Check sheet for the modelled part. Datum: model origin and axes. Units: mm. Face numbers are marked on the shaded views. A direction names the side the tool comes from. Coordinates: 2 decimals unless noted, no trailing zeros. Write each loop counter-clockwise with the first axis right and the second up, starting at its lowest first coordinate (ties: lowest second). Pieces come first, ordered by that corner, then holes. Notation, with made-up numbers: (9.5, -13) - (56.5, -13) arc R19 ccw to (56.5, 21) - close; hole circle Ø3 at (54.25, -20.5). An arc over 180 degrees is marked (long way). Write each question's results on one line, items separated by ' | '.
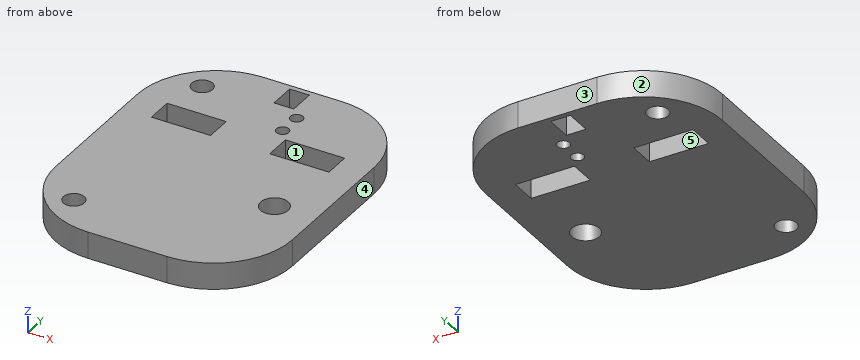
Autodesk Inventor part; units mm, degrees
ref_plane "YZ Plane" through (0, 0, 0) normal (1, 0, 0) x (0, 1, 0)
ref_plane "XZ Plane" through (0, 0, 0) normal (0, 1, 0) x (-1, 0, 0)
ref_plane "XY Plane" through (0, 0, 0) normal (0, 0, 1) x (1, 0, 0)
sketch "Sketch1" plane through (0, 0, 0) normal (0, 0, 1) x (1, 0, 0)
  circle A0 centre (10.5, 65) radius 2.65
  circle A1 centre (10.5, 10) radius 2.65
  circle A2 centre (49.5, 30) radius 3.5
  line L0 (60, 75) -> (60, 0)
  line L1 (60, 0) -> (0, 0)
  line L2 (0, 0) -> (0, 75)
  line L3 (0, 75) -> (60, 75)
  point P0 (30, 75)
  dimension "d0" = 39
  dimension "d1" = 5.3
  dimension "d2" = 55
  dimension "d3" = 10
  dimension "d5" = 10.5
  dimension "d16" = 10.5
  dimension "d19" = 20
  dimension "d22" = 7
  dimension "d55" = 75
  dimension "d64" = 60
extrude "Extrusion1" add sketch "Sketch1" along normal blind 6.731
sketch "Sketch3" plane through (0, 0, 6.731) normal (0, 0, 1) x (1, 0, 0)
  line L0 (60, 0) -> (60, 75)
  line L1 (60, 75) -> (0, 75)
  line L2 (0, 75) -> (0, 0)
  line L3 (7.5, 55) -> (22.5, 55)
  line L4 (22.5, 55) -> (22.5, 48.269)
  line L5 (22.5, 48.269) -> (7.5, 48.269)
  line L6 (7.5, 48.269) -> (7.5, 55)
  line L7 (37.5, 55) -> (52.5, 55)
  line L8 (52.5, 55) -> (52.5, 48.269)
  line L9 (52.5, 48.269) -> (37.5, 48.269)
  line L10 (37.5, 48.269) -> (37.5, 55)
  line L11 (27.5, 73.731) -> (32.5, 73.731)
  line L12 (32.5, 73.731) -> (32.5, 67)
  line L13 (32.5, 67) -> (27.5, 67)
  line L14 (27.5, 67) -> (27.5, 73.731)
  circle A0 centre (35, 64) radius 1.588
  circle A1 centre (35, 58) radius 1.588
  line L15 (37.5, 55) -> (30, 55) construction
  line L16 (30, 55) -> (22.5, 55) construction
  point P0 (30, 67)
  dimension "d70" = 15
  dimension "d71" = 6.731
  dimension "d73" = 15
  dimension "d74" = 7.5
  dimension "d75" = 7.5
  dimension "d78" = 20
  dimension "d81" = 12
  dimension "d84" = 3.176
  dimension "d91" = 3
  dimension "d92" = 6
  dimension "d93" = 3
  dimension "d94" = 5
  dimension "d95" = 5
extrude "Extrusion3" cut sketch "Sketch3" against normal up to next
fillet "Fillet2" radius 20 2 edges at (60, 0, 3.3655) (0, 0, 3.3655)
fillet "Fillet2" radius 20 2 edges at (0, 75, 3.3655) (60, 75, 3.3655)
equation "\"d16\" = d5"
equation "\"d20\" = THICKB"
equation "\"THICKA\" = 3.175"
equation "\"THICKB\" = 6.731"
equation "\"THICKC\" = 12.7"
equation "\"BALLDIA\" = 12"
equation "\"MAGDIA\" = 9.5"
equation "\"THICKPLY\" = 5"
properties part number "Carriage_Frame"
1. Sectioned sample at A-A (y = 30). Record the cut outline in (x, z).
Values follow:
outline: (0, 0) - (46, 0) - (46, 6.73) - (0, 6.73) - close; (53, 0) - (60, 0) - (60, 6.73) - (53, 6.73) - close
2. Draft check along X on the marked faces 3, 4 and 5. Enter one of: pulls with the +X half, pulls with the -X half, needs draft (parallel to the pull), parting line crosses it, or undercut.
Values follow:
face 3: needs draft | face 4: pulls with the +X half | face 5: undercut
3. Sectioned sample at D-D (x = 10.5). Record the cut outline in (y, z).
Values follow:
outline: (2.4, 0) - (7.35, 0) - (7.35, 6.73) - (2.4, 6.73) - close; (12.65, 0) - (48.27, 0) - (48.27, 6.73) - (12.65, 6.73) - close; (55, 0) - (62.35, 0) - (62.35, 6.73) - (55, 6.73) - close; (67.65, 0) - (72.6, 0) - (72.6, 6.73) - (67.65, 6.73) - close
4. Access from +Z, -Z, +X, -X, +Y, -Y to the whole of each face (thin tool, end or side, straight path). Record for the marked faces 1 and 2.
Values follow:
face 1: +Z, -Z | face 2: +Z, -Z, -X, +Y
5. Sectioned sample at C-C (z = 5). Give the number of separate pieces and of enclosed holes in the cut face, then the cut area to 3 significant figures.
Values follow:
separate pieces: 1 | enclosed holes: 8 | area: 3,820 mm^2
6. Sectioned sample at B-B (x = 35). Record the cut outline in (y, z).
Values follow:
outline: (0, 0) - (56.41, 0) - (56.41, 6.73) - (0, 6.73) - close; (59.59, 0) - (62.41, 0) - (62.41, 6.73) - (59.59, 6.73) - close; (65.59, 0) - (75, 0) - (75, 6.73) - (65.59, 6.73) - close
7. Material ranges on L1, parallel to Y at x = 35, z = 2; L2, parallel to Y at x = 21.5, z = 1.75; L3, parallel to Y at x = 10.5, z = 4.5, recorded low to high. Write a range as [from, to].
Values follow:
L1: y = [0, 56.41], [59.59, 62.41], [65.59, 75] | L2: y = [0, 48.27], [55, 75] | L3: y = [2.4, 7.35], [12.65, 48.27], [55, 62.35], [67.65, 72.6]
8. Go/stop test with flat-tipped pins: pin 1 (8.5 mm diameter, centred on x = 10.5, y = 10, fed in from -Z); pin 2 (1 mm diameter, centred on y = 64.5, z = 2, fed in from -X); pin 3 (3 mm diameter, centred on x = 35, y = 58, fed in from -Z); pin 4 (3.5 mm diameter, centred on y = 71, z = 4.5, fed in from +X). Record where each tip stops, or that it passes through.
Values follow:
pin 1: stops at z = 0 | pin 2: stops at x = 2.14 | pin 3: passes through | pin 4: stops at x = 54.03
